Here's how the part is built. I have some questions about the finished solid (model axes, mm). Face numbers are marked on the shaded views. A direction names the side the tool comes from. Coordinates: 2 decimals unless noted, no trailing zeros. Write each loop counter-clockwise with the first axis right and the second up, starting at its lowest first coordinate (ties: lowest second). Pieces come first, ordered by that corner, then holes.
from build123d import *

# Parameters (mm, degrees)
F0_W     = 2.54
F0_H     = 225.552
F1_DEPTH = 143.256
F2_W     = 25.4
F2_H     = 30.48
F3_DEPTH = 143.256
F4_W     = 25.4
F4_H     = 25.4
F5_DEPTH = 177.8


with BuildPart() as f1:
    # F0 (on Front) → F1 (new body)
    with BuildSketch(Plane.XZ):
        with Locations((-19.223887, 91.398376)):
            Rectangle(F0_W, F0_H)
    extrude(amount=F1_DEPTH)

    # F2 (on face) → F3 (join)
    with BuildSketch(Plane.XZ.offset(143.256)):
        with Locations((-33.193887, 105.114376)):
            Rectangle(F2_W, F2_H)
    extrude(amount=-F3_DEPTH)

    # F4 (on face) → F5 (cut)
    with BuildSketch(Plane.XZ.offset(143.256)):
        with Locations((-30.653887, 105.114376)):
            Rectangle(F4_W, F4_H)
    extrude(amount=-F5_DEPTH, mode=Mode.SUBTRACT)


solid = f1.part
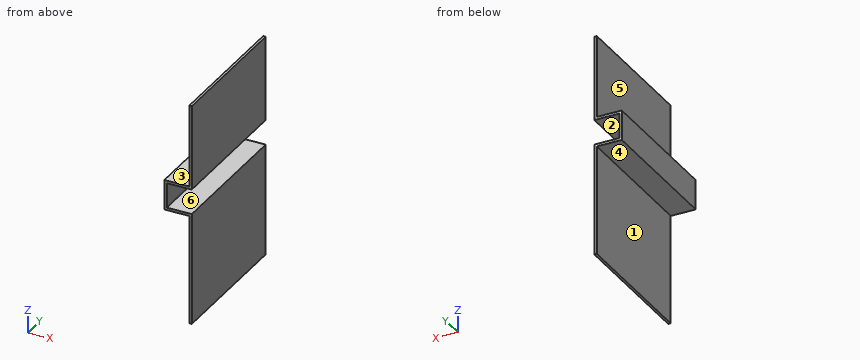
1. If I drill on line 1 (Z direction, x = -41, y = -37.5); line 2 (Z direction, x = -19.25, y = -58); line 3 (X direction, y = -64.5, z = 145), over which ranges is the centre line in solid material (lowest first)?
2. I want a section at A-A (x = -39.75). List the corners of the cut face in (y, z) for me, then the cut area to 3 significant figures.
3. I want a section at B-B (y = -36.5). List the corners of the cut face in (x, z) for me.
4. I want a section at C-C (z = 66.5). List the corners of the cut face in (x, y) for me, then the cut area to 3 significant figures.
5. Thinking about a two-plate mould opening in Z: for the marked faces 4, 5 and 6, which applies, pulls with the +Z half, pulls with the -Z half, needs draft (parallel to the pull), parting line crosses it, or undercut?
6. On a 3-axis mill with a long thin cutter (end or side, diameter ignored), from which of +Z, -Z, +X, -X, +Y, -Y can I reach the whole of each face in a straight line? I mean the marked faces 1, 2 and 3. Say none if no direction works.
7. For pin 1 Ø7.5 at (x, y) = (-27, -37.5) entering from -Z; pin 2 Ø7.5 at (y, z) = (-45.5, 100) entering from +X; pin 3 Ø2 at (x, y) = (-42.5, -62.5) entering from +Z; pin 4 Ø12 at (x, z) = (-26, 133.5) entering from +Y, each with a flat end and sliding along its axis, tell me the tip position at first contact or that it passes through.
Response values:
1. line 1: z = 89.87 to 92.41, 117.81 to 120.35
1. line 2: z = -21.38 to 92.41, 117.81 to 204.17
1. line 3: x = -20.49 to -17.95
2. outline: (-143.26, 89.87) - (0, 89.87) - (0, 92.41) - (-143.26, 92.41) - close; (-143.26, 117.81) - (0, 117.81) - (0, 120.35) - (-143.26, 120.35) - close
2. area: 728 mm2
3. outline: (-45.89, 89.87) - (-20.49, 89.87) - (-20.49, -21.38) - (-17.95, -21.38) - (-17.95, 92.41) - (-43.35, 92.41) - (-43.35, 117.81) - (-17.95, 117.81) - (-17.95, 204.17) - (-20.49, 204.17) - (-20.49, 120.35) - (-45.89, 120.35) - close
4. outline: (-20.49, -143.26) - (-17.95, -143.26) - (-17.95, 0) - (-20.49, 0) - close
4. area: 364 mm2
5. face 4: pulls with the -Z half
5. face 5: needs draft
5. face 6: undercut
6. face 1: -Z, -X, +Y, -Y
6. face 2: +X, +Y, -Y
6. face 3: +Z, -X, +Y, -Y
7. pin 1: stops at z = 89.87
7. pin 2: stops at x = -43.35
7. pin 3: stops at z = 120.35
7. pin 4: stops at y = 0
